Geometry check sheet. Reference: the model listing, model coordinates, mm. A direction names the side the tool comes from. Round coordinates to 2 decimals unless told otherwise and drop trailing zeros. Write each loop counter-clockwise with the first axis right and the second up, starting at its lowest first coordinate (ties: lowest second). Pieces come first, ordered by that corner, then holes. Notation, with made-up numbers: M 66,74 L 104,74 A22 ccw 104,85 Z; hole C -15,-11.75 d11. An arc over 180 degrees is marked long. Put each result on its own line as item: value. Start each with the question number.
(1) Section check C-C on y = 60. Record the cut outline in (x, z), then the cut area to 3 significant figures.
(2) Section check D-D on y = 30. Record the cut outline in (x, z).
(3) Section check A-A on x = 0. Record the cut outline in (y, z), then the cut area to 3 significant figures.
(4) Material ranges on probe 1 along X at (y, z) = (101.5, 1.2); probe 2 along X at (y, z) = (77, 0.3); probe 3 along X at (y, z) = (61, 1.4), recorded low to high.
(5) Section check B-B on z = 1.3. Record the cut outline in (x, y), then the cut area to 3 significant figures.
(6) Mould release check, pull along Y, two halves, no side actions. Record for faces 4 (the cylindrical face through (-25.5, 75.5, 1.5)), 5 (the cylindrical face through (26.99, 114.15, 1.48)), 6 (the flat face through (-9, 81, 0)): pulls with the +Y half, pulls with the -Y half, needs draft (parallel to the pull), parting line crosses it, or undercut.
(7) Tool access check on faces 1 (the cylindrical face through (0.14, 37.9, 1.48)), 2 (the flat face through (30, 86, 1)), 3 (the flat face through (-30, 86, 1)). Record the directions out of +Z, -Z, +X, -X, +Y, -Y that give a thin tool (end or side, any length) a straight path to the whole face; none if there is none.
(8) Gauge pin test, flat ends, axial feed: pin 1 (1.5 mm diameter, centred on y = 83.5, z = 1.5, fed in from +X); pin 2 (12 mm diameter, centred on x = -26.5, y = 36, fed in from +Z); pin 3 (3.5 mm diameter, centred on x = -8, y = 30, fed in from -Z); pin 4 (1.5 mm diameter, centred on y = 62, z = 1.5, fed in from +X). Record the tip position at first contact, or that the pin passes through.
from build123d import *

# Parameters (mm, degrees)
SKETCH_1_R      = 1.5
EXTRUDE_1_DEPTH = 3


with BuildPart() as part:
    # 草图1 → 凸台-拉伸1 (new body)
    with BuildSketch(Plane.XY):
        with BuildLine():
            Line((30, 65), (43.229490169, 55))
            ThreePointArc((43.229490169, 55), (24.322951332, 45.093216766), (10.332713198, 28.972583968))
            ThreePointArc((10.332713198, 28.972583968), (0, 23.037780053), (-10.332713198, 28.972583968))
            ThreePointArc((-10.332713198, 28.972583968), (-24.322951332, 45.093216766), (-43.229490169, 55))
            Line((-43.229490169, 55), (-30, 65))
            Line((-30, 65), (-30, 107))
            ThreePointArc((-30, 107), (-27.071067812, 114.071067812), (-20, 117))
            Line((-20, 117), (20, 117))
            ThreePointArc((20, 117), (27.071067812, 114.071067812), (30, 107))
            Line((30, 107), (30, 65))
        make_face()
        with Locations((-30, 60)):
            Circle(SKETCH_1_R, mode=Mode.SUBTRACT)
        with Locations((-8, 30)):
            Circle(SKETCH_1_R, mode=Mode.SUBTRACT)
        with Locations((8, 30)):
            Circle(SKETCH_1_R, mode=Mode.SUBTRACT)
        with Locations((30, 60)):
            Circle(SKETCH_1_R, mode=Mode.SUBTRACT)
        with BuildLine():
            Line((27, 102), (27, 77))
            ThreePointArc((27, 77), (25.5, 75.5), (24, 77))
            Line((24, 77), (24, 102))
            ThreePointArc((24, 102), (25.5, 103.5), (27, 102))
        make_face(mode=Mode.SUBTRACT)
        with BuildLine():
            Line((-27, 102), (-27, 77))
            ThreePointArc((-27, 77), (-25.5, 75.5), (-24, 77))
            Line((-24, 77), (-24, 102))
            ThreePointArc((-24, 102), (-25.5, 103.5), (-27, 102))
        make_face(mode=Mode.SUBTRACT)
        with BuildLine():
            Line((-6.54179371, 44.438430627), (-6.54179371, 93.748949186))
            ThreePointArc((-6.54179371, 93.748949186), (0, 100.290742896), (6.54179371, 93.748949186))
            Line((6.54179371, 93.748949186), (6.54179371, 44.438430627))
            ThreePointArc((6.54179371, 44.438430627), (0, 37.896636917), (-6.54179371, 44.438430627))
        make_face(mode=Mode.SUBTRACT)
    extrude(amount=EXTRUDE_1_DEPTH)


solid = part.part
Answers follow:
1. outline: M -36.61,0 L -31.5,0 L -31.5,3 L -36.61,3 Z; M -28.5,0 L -6.54,0 L -6.54,3 L -28.5,3 Z; M 6.54,0 L 28.5,0 L 28.5,3 L 6.54,3 Z; M 31.5,0 L 36.61,0 L 36.61,3 L 31.5,3 Z
1. area: 162 mm^2
2. outline: M -10.95,0 L -9.5,0 L -9.5,3 L -10.95,3 Z; M -6.5,0 L 6.5,0 L 6.5,3 L -6.5,3 Z; M 9.5,0 L 10.95,0 L 10.95,3 L 9.5,3 Z
3. outline: M 23.04,0 L 37.9,0 L 37.9,3 L 23.04,3 Z; M 100.29,0 L 117,0 L 117,3 L 100.29,3 Z
3. area: 94.7 mm^2
4. probe 1: x = -30 to -27, -24 to 24, 27 to 30
4. probe 2: x = -30 to -27, -24 to -6.54, 6.54 to 24, 27 to 30
4. probe 3: x = -35.29 to -31.12, -28.88 to -6.54, 6.54 to 28.88, 31.12 to 35.29
5. outline: M -43.23,55 A57.5 cw -10.33,28.97 A11.96 ccw 10.33,28.97 A57.5 cw 43.23,55 L 30,65 L 30,107 A10 ccw 20,117 L -20,117 A10 ccw -30,107 L -30,65 Z; hole C -30,60 d3; hole M -27,77 A1.5 ccw -24,77 L -24,102 A1.5 ccw -27,102 Z; hole C -8,30 d3; hole M -6.54,44.44 A6.54 ccw 6.54,44.44 L 6.54,93.75 A6.54 ccw -6.54,93.75 Z; hole C 8,30 d3; hole M 24,77 A1.5 ccw 27,77 L 27,102 A1.5 ccw 24,102 Z; hole C 30,60 d3
5. area: 4,100 mm^2
6. face 4: undercut
6. face 5: pulls with the +Y half
6. face 6: needs draft
7. face 1: +Z, -Z
7. face 2: +Z, -Z, +X, +Y
7. face 3: +Z, -Z, -X, +Y
8. pin 1: stops at x = 30
8. pin 2: passes through
8. pin 3: stops at z = 0
8. pin 4: stops at x = 34.96
